Geometry check sheet. Reference: the model listing, model coordinates, mm. Face numbers are marked on the shaded views. A direction names the side the tool comes from. Coordinates: 2 decimals unless noted, no trailing zeros. Write each loop counter-clockwise with the first axis right and the second up, starting at its lowest first coordinate (ties: lowest second). Pieces come first, ordered by that corner, then holes. Notation, with made-up numbers: (-19.75, 21.25) -> (15.25, 21.25) arc R16 cw to (15.25, 26.25) -> close; hole circle Ø3 at (45.5, 44). An arc over 180 degrees is marked (long way). One line per question, with ' | ' between items.
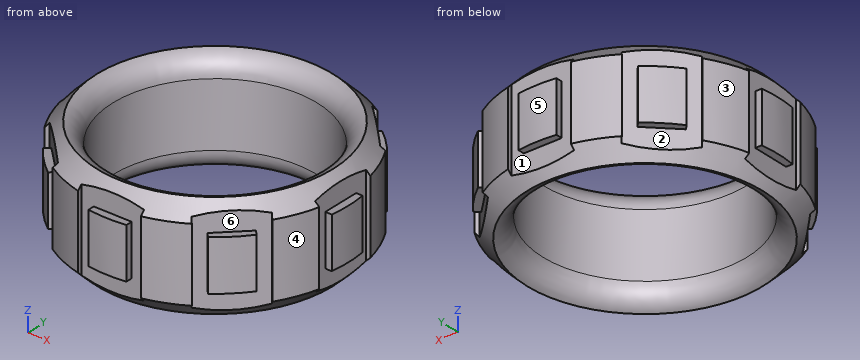
```python
from build123d import *

# Parameters (mm, degrees)
F0_R            = 12.75
F0_R_2          = 9.75
F1_DEPTH        = 10
F2_SIZE         = 1.5
F4_W            = 6
F4_H            = 10
F4_W_2          = 3.618944902
F4_H_2          = 4.83566802
F5_DEPTH        = 2
F5_COPIES_COUNT = 8


# Not quite as in the source:
# - a fillet or chamfer that OpenCascade refuses, or shapes differently, is made with other operations: its cross-section is extruded or revolved along the edge and cut away or added
# - a pattern or mirror of a feature is missing from the dataset's text; its kind, count and spacing are read off the source's solid


with BuildPart() as f1:
    # F0 (on Top) → F1 (new body)
    with BuildSketch(Plane.XY):
        Circle(F0_R)
        Circle(F0_R_2, mode=Mode.SUBTRACT)
    extrude(amount=F1_DEPTH)

    # F2
    f2_edges = [f1.edges().sort_by_distance(p)[0] for p in [
        (-12.75, 0, 10),
        (-12.75, 0, 0),
    ]]
    chamfer(f2_edges, length=F2_SIZE)

    # F4 (on offset) → F5 (cut)
    with BuildSketch(Plane.YZ.offset(14)):
        with Locations((0, 5.0058439374)):
            Rectangle(F4_W, F4_H)
        with Locations((0, 5.0058439374)):
            Rectangle(F4_W_2, F4_H_2, mode=Mode.SUBTRACT)
    f5 = extrude(amount=-F5_DEPTH, mode=Mode.SUBTRACT)

    # F5_copies: F5 ×8 about axis
    f5_copies_axis = Axis((0, 0, 0), (0, 0, 1))
    for i in range(1, F5_COPIES_COUNT):
        add(f5.rotate(f5_copies_axis, i * 360 / F5_COPIES_COUNT), mode=Mode.SUBTRACT)

    # F6: fillet of radius 2 on 2 edges, made by hand

    # F6_s1 → F6_t2 (revolve, cut)
    with BuildSketch(Plane.XZ):
        with BuildLine():
            ThreePointArc((11.25, 10), (10.1688611699, 9.2882531983), (9.75, 8.0635083269))
            Line((9.75, 8.0635083269), (9.75, 10))
            Line((9.75, 10), (11.25, 10))
        make_face()
    revolve(axis=Axis((0, 0, 10), (0, 0, 1)), mode=Mode.SUBTRACT)

    # F6_s3 → F6_t4 (revolve, cut)
    with BuildSketch(Plane.XZ):
        with BuildLine():
            ThreePointArc((11.25, 0), (10.1688611699, 0.7117468017), (9.75, 1.9364916731))
            Line((9.75, 1.9364916731), (9.75, 0))
            Line((9.75, 0), (11.25, 0))
        make_face()
    revolve(axis=Axis((0, 0, 0), (0, 0, 1)), mode=Mode.SUBTRACT)


solid = f1.part
```
(1) Draft check along X on the marked faces 1, 2, 3 and 4. Enter one of: pulls with the +X half, pulls with the -X half, needs draft (parallel to the pull), parting line crosses it, or undercut.
Answers below:
face 1: undercut | face 2: undercut | face 3: pulls with the -X half | face 4: pulls with the +X half
(2) Material ranges on line 1 (X direction, y = 0.25, z = 3); line 2 (X direction, y = 7.5, z = 7.5); line 3 (Y direction, x = -10, z = 4.75), recorded low to high.
Answers below:
line 1: x = -12.75 to -9.75, 9.75 to 12.75 | line 2: x = -9.47 to -6.23, 6.23 to 9.47 | line 3: y = -7.91 to -7.44, -6.97 to 6.97, 7.44 to 7.91
(3) Depth check by flat-ended pin: P1, Ø1.5, axis at x = 9, y = 8, coming from the -Z side; P2, Ø4, axis at y = -6, z = 6, coming from the -X side; P3, Ø4, axis at y = -9, z = 2, coming from the -X side; P4, Ø1.5, axis at x = -0.5, y = 7.5, coming from the -Z side. Enter the tip coordinate at first touch or a pass-through.
Answers below:
P1: stops at z = 0.04 | P2: stops at x = -12.11 | P3: stops at x = -10.2 | P4: passes through
(4) Tool access check on the marked faces 5 and 6. Record the directions out of +Z, -Z, +X, -X, +Y, -Y that give a thin tool (end or side, any length) a straight path to the whole face; none if there is none.
Answers below:
face 5: +Z, -Z, +Y | face 6: none
(5) Cross-section at A-A (x = 0). Record the cut outline in (y, z), plus the area to 3 significant figures.
Answers below:
outline: (-12.75, 2.59) -> (-12, 2.59) -> (-12, 0.75) -> (-11.25, 0) arc R2 ccw to (-9.75, 1.94) -> (-9.75, 8.06) arc R2 ccw to (-11.25, 10) -> (-12, 9.25) -> (-12, 7.42) -> (-12.75, 7.42) -> close; (9.75, 1.94) arc R2 ccw to (11.25, 0) -> (12, 0.75) -> (12, 2.59) -> (12.75, 2.59) -> (12.75, 7.42) -> (12, 7.42) -> (12, 9.25) -> (11.25, 10) arc R2 ccw to (9.75, 8.06) -> close | area: 48.1 mm²
